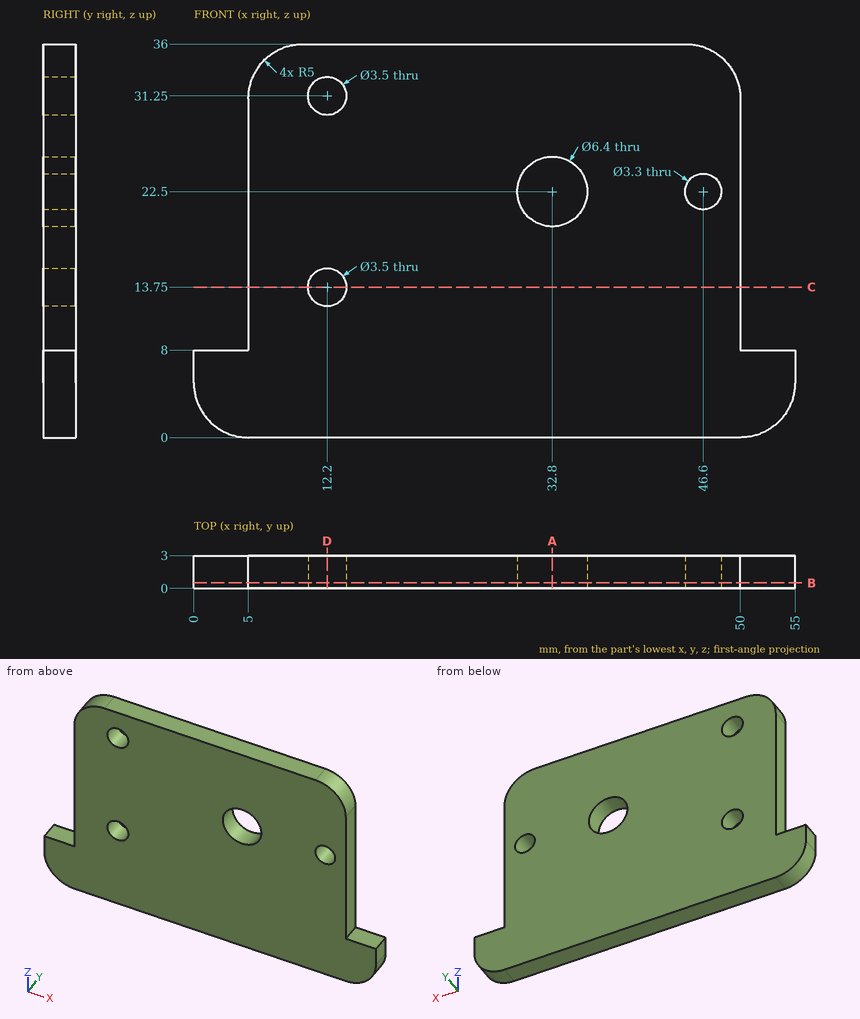
The drawing under review shows one solid part. Ordinate dimensions are in mm from its lowest x, y, z. Round coordinates to 2 decimals unless told otherwise and drop trailing zeros. Write each loop counter-clockwise with the first axis right and the second up, starting at its lowest first coordinate (ties: lowest second). Pieces come first, ordered by that corner, then holes. Notation, with made-up numbers: M 86.25,-20.5 L 127.25,-20.5 A30 cw 127.25,8.5 Z; hole C -25,-21.5 d4. An arc over 180 degrees is marked long. One line per item, written item: value. Start each with the question number.
(1) We need section D-D (x = 12.2). Give the boundary of the cut face in (y, z), and give its area (3 significant figures).
(2) Insertion check: pin 1 (3 mm diameter, centred on x = 12.2, z = 13.75, fed in from -Y); pin 2 (0.9 mm diameter, centred on x = 2.5, y = 1.5, fed in from +Z); pin 3 (1 mm diameter, centred on y = 2, z = 32, fed in from +X). Each pin has a flat end and moves straight along its axis. Give the tip position at first contact, or say it passes through.
(3) We need section C-C (z = 13.75). Give the boundary of the cut face in (x, y).
(4) Wall thickness on line 1 (X direction, y = 1.85, z = 22.5); line 2 (X direction, y = 0.7, z = 13.75); line 3 (X direction, y = 0.3, z = 13): over which ranges is each line inside the solid? List them lowest first.
(5) We need section B-B (y = 0.5). Give the boundary of the cut face in (x, z).
(6) We need section A-A (x = 32.8). Give the boundary of the cut face in (y, z), and give its area (3 significant figures).
Result:
1. outline: M 0,0 L 3,0 L 3,12 L 0,12 Z; M 0,15.5 L 3,15.5 L 3,29.5 L 0,29.5 Z; M 0,33 L 3,33 L 3,36 L 0,36 Z
1. area: 87.0 mm²
2. pin 1: through
2. pin 2: z = 8
2. pin 3: x = 49.97
3. outline: M 5,0 L 10.45,0 L 10.45,3 L 5,3 Z; M 13.95,0 L 50,0 L 50,3 L 13.95,3 Z
4. line 1: 5 to 29.6, 36 to 44.95, 48.25 to 50
4. line 2: 5 to 10.45, 13.95 to 50
4. line 3: 5 to 10.62, 13.78 to 50
5. outline: M 0,5 A5 ccw 5,0 L 50,0 A5 ccw 55,5 L 55,8 L 50,8 L 50,31 A5 ccw 45,36 L 10,36 A5 ccw 5,31 L 5,8 L 0,8 Z; hole C 12.2,13.75 d3.5; hole C 12.2,31.25 d3.5; hole C 32.8,22.5 d6.4; hole C 46.6,22.5 d3.3
6. outline: M 0,0 L 3,0 L 3,19.3 L 0,19.3 Z; M 0,25.7 L 3,25.7 L 3,36 L 0,36 Z
6. area: 88.8 mm²
